from build123d import *

# Parameters (mm, degrees)
F0_R     = 11.938
F0_R_2   = 6.7437
F1_DEPTH = 15.24
F2_DEPTH = 1.016
F4_DEPTH = 48.26
F5_R     = 25.39999
F6_R     = 12.7
F7_DEPTH = 25.4
F8_R     = 3.175
F9_DEPTH = 13.1042779754


# Not quite as in the source:
# - a fillet or chamfer is up to 0.001 mm smaller than in the source, because OpenCascade refuses the exact size
# - a feature names something its author has since deleted; it is built from what else it names


with BuildPart() as f1:
    # F0 (on Top) → F1 (new body)
    with BuildSketch(Plane.XY):
        with BuildLine():
            Line((44.45, 25.4), (-44.45, 25.4))
            ThreePointArc((-44.45, 25.4), (-69.85, 0), (-44.45, -25.4))
            Line((-44.45, -25.4), (44.45, -25.4))
            ThreePointArc((44.45, -25.4), (69.85, 0), (44.45, 25.4))
        make_face()
        with Locations((-44.45, 0)):
            Circle(F0_R, mode=Mode.SUBTRACT)
        Polygon((-12.1442471439, -24.5133200793), (-25.6998479864, -9.3756820272), (12.1442471439, 24.5133200793), (25.6998479864, 9.3756820272), align=None, mode=Mode.SUBTRACT)
        with Locations((44.45, 0)):
            Circle(F0_R, mode=Mode.SUBTRACT)
        with Locations((-44.45, 0)):
            Circle(F0_R)
        with Locations((-44.45, 0)):
            Circle(F0_R_2, mode=Mode.SUBTRACT)
        with Locations((44.45, 0)):
            Circle(F0_R)
        with Locations((44.45, 0)):
            Circle(F0_R_2, mode=Mode.SUBTRACT)
        Polygon((12.1442471439, 24.5133200793), (-25.6998479864, -9.3756820272), (-12.1442471439, -24.5133200793), (25.6998479864, 9.3756820272), align=None)
    extrude(amount=-F1_DEPTH)

    # F0 (on Top) → F2 (cut)
    with BuildSketch(Plane.XY):
        with Locations((-44.45, 0)):
            Circle(F0_R)
        with Locations((-44.45, 0)):
            Circle(F0_R_2, mode=Mode.SUBTRACT)
        with Locations((44.45, 0)):
            Circle(F0_R)
        with Locations((44.45, 0)):
            Circle(F0_R_2, mode=Mode.SUBTRACT)
    extrude(amount=-F2_DEPTH, mode=Mode.SUBTRACT)

    # F0 (on Top) → F4 (join)
    with BuildSketch(Plane.XY):
        Polygon((12.1442471439, 24.5133200793), (-25.6998479864, -9.3756820272), (-12.1442471439, -24.5133200793), (25.6998479864, 9.3756820272), align=None)
    extrude(amount=F4_DEPTH)

    # F5 (radius 25.4 in the source; OpenCascade refuses exactly that, so slightly less here)
    f5_edges = [f1.edges().sort_by_distance(p)[0] for p in [
        (-18.922048, -16.944501, 48.26),
        (18.922048, 16.944501, 48.26),
    ]]
    fillet(f5_edges, radius=F5_R)

    # F6 (on face) → F7 (cut)
    with BuildSketch(Plane(origin=(6.7778004213, -7.5688190261, 0), x_dir=(0.7449625026, 0.6671063407, 0), z_dir=(0.6671063407, -0.7449625026, 0))):
        with Locations((0, 22.86)):
            Circle(F6_R)
    extrude(amount=-F7_DEPTH, mode=Mode.SUBTRACT)

    # F8 (on offset) → F9 (cut, through all)
    with BuildSketch(Plane.XY.offset(48.26)):
        Circle(F8_R)
    extrude(amount=-F9_DEPTH, mode=Mode.SUBTRACT)


solid = f1.part
Geometry: final body of the model. Coordinates: model frame, mm. A direction names the side the tool comes from. Give positions to 0.01 mm unless a question says otherwise; leave off trailing zeros. Write each loop counter-clockwise with the first axis right and the second up, starting at its lowest first coordinate (ties: lowest second). Pieces come first, ordered by that corner, then holes. Notation, with made-up numbers: (-28.5, 84.5) -> (9.5, 84.5) arc R24 cw to (9.5, 100.5) -> close; hole circle Ø11 at (29.25, 8.25). An arc over 180 degrees is marked (long way). Answer as a JSON object with one key per item and string values.
1. Cut plane D-D on y = -5. Count the separate pieces of the cut face and the enclosed holes in it, and give its area (3 significant figures).
Ans:
{"separate pieces": "3", "enclosed holes": "0", "area": "2,750 mm^2"}
2. Contact query for flat-ended pins moving along their axis: pin 1 (1.5 mm diameter, centred on x = 42, y = -10.5, fed in from +Z); pin 2 (1 mm diameter, centred on y = 6, z = 19, fed in from -X); pin 3 (3 mm diameter, centred on x = -8, z = 2, fed in from -Y). Output: stop coordinate, or through.
Ans:
{"pin 1": "stops at z = -1.02", "pin 2": "stops at x = 10.37", "pin 3": "stops at y = -22.15"}
3. Mould query, pull axis X, two halves, no side actions, for faces 5 (the flat face through (-39, -5, -1.016)), 6 (the cylindrical face through (-49.42, 4.56, -8.03)), 7 (the flat face through (-17, 0, 0)), 8 (the cylindrical face through (69.844, -0.559, -7.513)). Classes: pulls with the +X half, pulls with the -X half, needs draft (parallel to the pull), parting line crosses it, or undercut.
Ans:
{"face 5": "undercut", "face 6": "undercut", "face 7": "needs draft", "face 8": "pulls with the +X half"}
4. Access query for faces 1 (the flat face through (-1.9, -15.34, 29.15)), 2 (the flat face through (1.9, 15.34, 29.15)), 3 (the flat face through (19.017, 16.839, 11.27)), 4 (the flat face through (50, -5, -1.016)). Directions: +Z, -Z, +X, -X, +Y, -Y. A direction counts if a zero-diameter tool reaches every point of the face in a straight line with its end or side. Return the directions, or none.
Ans:
{"face 1": "+Z, +X, -Y", "face 2": "+Z, -X, +Y", "face 3": "+Z, +X, +Y", "face 4": "+Z"}
5. Cut plane A-A on z = 20. Output: boundary loops of the cut face in (x, y), and give its area (3 significant figures).
Ans:
{"outline": "(-25.7, -9.38) -> (-12.14, -24.51) -> (-2.44, -15.82) -> (-16, -0.69) -> close; (2.44, 15.82) -> (16, 0.69) -> (25.7, 9.38) -> (12.14, 24.51) -> close", "area": "529 mm^2"}
6. Cut plane B-B on z = -11. Output: boundary loops of the cut face in (x, y).
Ans:
{"outline": "(-44.45, -25.4) -> (44.45, -25.4) arc R25.4 ccw to (44.45, 25.4) -> (-44.45, 25.4) arc R25.4 ccw to start; hole circle Ø13.49 at (-44.45, 0); hole circle Ø13.49 at (44.45, 0)"}
7. Cut plane C-C on x = -41. Output: boundary loops of the cut face in (y, z).
Ans:
{"outline": "(-25.4, -15.24) -> (-5.79, -15.24) -> (-5.79, -1.02) -> (-11.43, -1.02) -> (-11.43, 0) -> (-25.4, 0) -> close; (5.79, -15.24) -> (25.4, -15.24) -> (25.4, 0) -> (11.43, 0) -> (11.43, -1.02) -> (5.79, -1.02) -> close"}
8. Ray query, probe 1 along Y at (x, z) = (-44.45, -5.75); probe 2 along Z at (x, y) = (-60.5, 13); probe 3 along Z at (x, y) = (-0.5, 7). Return the intervals inside material, ascending. Write a range as from..to.
Ans:
{"probe 1": "y = -25.4..-6.74, 6.74..25.4", "probe 2": "z = -15.24..0", "probe 3": "z = -15.24..10.91, 34.81..47.89"}
